Could you check a few things on this model? Use its own coordinates, in mm. A direction names the side the tool comes from. Round coordinates to 2 decimals unless told otherwise and drop trailing zeros. Write each loop counter-clockwise with the first axis right and the second up, starting at its lowest first coordinate (ties: lowest second). Pieces come first, ordered by that corner, then holes. Notation, with made-up numbers: M 22,72.25 L 67,72.25 A15 cw 67,85.25 Z; hole C 29,49.5 d9. An arc over 180 degrees is marked long. One line per item, written item: value. Start each with the question number.
(1) I want a section at D-D on x = 5. Please give me the cut outline in (y, z).
(2) I want a section at A-A on y = 23. Please give me the cut outline in (x, z).
(3) Thinking about a two-plate mould opening in Z: for faces 1 (the face through (27, 16, -15)), 2 (the face through (14, 15, 0)), 3 (the face through (29, 15, -14)), 4 (the face through (15, 15, -29)), which applies, released by +Z, released by -Z, zero draft, split by the parting line, or undercut?
(4) I want a section at C-C on z = -4.5. Please give me the cut outline in (x, y), and give its area (3 significant figures).
(5) I want a section at B-B on x = 26. Please give me the cut outline in (y, z).
(6) I'm going to push flat-ended pins straight in: pin 1 Ø3 at (x, y) = (5, 5) entering from +Z; pin 2 Ø1 at (x, z) = (18.5, -20.5) entering from +Y. Where does each tip first touch, or does it pass through?
(7) If I drill on L1, parallel to X at y = 13, z = -2.25; L2, parallel to Y at x = 5, z = -0.6; L3, parallel to Z at x = 15, y = 26, over which ranges is the centre line in solid material (lowest first)?
(8) Which directions (+Z, -Z, +X, -X, +Y, -Y) give clear straight access to the entire face, cutting with the end or side of a thin tool? Please do faces 5 (the face through (14, 2, -15)), 6 (the face through (28, 30, -14)), 7 (the face through (3, 5, -1)).
Autodesk Inventor part; units mm, degrees
ref_plane "YZ Plane" through (0, 0, 0) normal (1, 0, 0) x (0, 1, 0)
ref_plane "XZ Plane" through (0, 0, 0) normal (0, 1, 0) x (-1, 0, 0)
ref_plane "XY Plane" through (0, 0, 0) normal (0, 0, 1) x (1, 0, 0)
sketch "Sketch7" plane through (0, 0, 0) normal (0, 1, 0) x (-1, 0, 0)
  point P0 (0, 0)
sketch "Sketch8" plane through (0, 0, 0) normal (0, 1, 0) x (-1, 0, 0)
  line L0 (0, 0) -> (-29, 0)
  line L1 (-29, 0) -> (-29, -29)
  line L2 (-29, -29) -> (0, -29)
  line L3 (0, -29) -> (0, 0)
  line L4 (-2, -27) -> (-27, -27)
  line L5 (-27, -27) -> (-27, -2)
  line L6 (-27, -2) -> (-2, -2)
  line L7 (-2, -2) -> (-2, -27)
  dimension "d25" = 29
  dimension "d26" = 29
  dimension "d38" = 2
extrude "Extrusion5" add sketch "Sketch8" along normal blind 30 contours L3 L2 L1 L0 | L4 L5 L6 L7
sketch "Sketch11" plane through (0, 30, 0) normal (0, 1, 0) x (1, 0, 0)
  line L0 (0, 0) -> (29, 0)
  line L1 (29, 0) -> (29, 29)
  line L2 (29, 29) -> (0, 29)
  line L3 (0, 29) -> (0, 0)
  line L4 (2, 27) -> (27, 27)
  line L5 (27, 27) -> (27, 2)
  line L6 (27, 2) -> (2, 2)
  line L7 (2, 2) -> (2, 27)
  dimension "d39" = 2
extrude "Extrusion8" cut sketch "Sketch11" against normal blind 28 contours L4 L5 L6 L7
sketch "Sketch12" plane through (0, 0, 0) normal (0, 0, 1) x (1, 0, 0)
  line L0 (2, 30) -> (27, 30)
  line L1 (2, 30) -> (2, 2)
  line L2 (27, 30) -> (27, 2)
  line L3 (2, 2) -> (5, 2)
  line L4 (5, 2) -> (5, 5)
  line L5 (5, 5) -> (2, 5)
  line L6 (2, 5) -> (2, 2)
  circle A0 centre (5, 5) radius 2
  line L7 (2, 2) -> (27, 2)
  point P0 (0, 0)
  dimension "d42" = 3
  dimension "d43" = 3
  dimension "d44" = 4
extrude "Extrusion9" cut sketch "Sketch12" against normal blind 2 contours A0 L4 L5 | L5 L4 A0
equation "\"BendRadius\" = Thickness"
equation "\"BendReliefWidth\" = Thickness"
equation "\"BendReliefDepth\" = 0.5 * Thickness"
equation "\"CornerReliefSize\" = 4 * Thickness"
equation "\"MinimumRemnant\" = 2 * Thickness"
equation "\"TransitionRadius\" = BendRadius"
equation "\"JacobiRadiusSize\" = Thickness"
equation "\"GapSize\" = Thickness"
properties part number "waterBallonHolderv2"
Found:
1. outline: M 0,-29 L 30,-29 L 30,-27 L 2,-27 L 2,-2 L 3,-2 L 3,0 L 0,0 Z; M 7,-2 L 30,-2 L 30,0 L 7,0 Z
2. outline: M 0,-29 L 29,-29 L 29,0 L 0,0 Z; hole M 2,-27 L 27,-27 L 27,-2 L 2,-2 Z
3. face 1: undercut
3. face 2: released by +Z
3. face 3: zero draft
3. face 4: released by -Z
4. outline: M 0,0 L 29,0 L 29,30 L 27,30 L 27,2 L 2,2 L 2,30 L 0,30 Z
4. area: 170 mm²
5. outline: M 0,-29 L 30,-29 L 30,-27 L 2,-27 L 2,-2 L 30,-2 L 30,0 L 0,0 Z
6. pin 1: stops at z = -27
6. pin 2: stops at y = 2
7. L1: x = 0 to 2, 27 to 29
7. L2: y = 0 to 3, 7 to 30
7. L3: z = -29 to -27, -2 to 0
8. face 5: +Y
8. face 6: +Z, -Z, +X, -X, +Y
8. face 7: +Z
